Build history of the part. All positions in model axes, mm. Face numbers are marked on the shaded views. Give positions to 0.01 mm unless a question says otherwise; leave off trailing zeros. Loops run counter-clockwise (first coordinate to the right, second up) from the corner with the lowest first, then second, coordinate; pieces in that order, holes last. Notation, with made-up numbers: (80.5, 33) -> (87.5, 33) arc R28 cw to (87.5, 62) -> close; hole circle Ø10 at (31.5, 25). An arc over 180 degrees is marked (long way). One line per question, with ' | ' between items. Start each with the question number.
(1) Drill centre lines: L1, parallel to Y at x = -24, z = 6.5; L2, parallel to Y at x = -37.5, z = 11; L3, parallel to X at y = 22, z = 8.25. Where is each one in solid material? Low to high. Write a range as from..to.
(2) Mould opens along Y. For the marked faces 1, 2 and 3 say: pulls with the +Y half, pulls with the -Y half, needs draft (parallel to the pull), parting line crosses it, or undercut.
(3) Slice it at C-C, the plane y = 20. Write the cut outline in (x, z), then the cut area to 3 significant figures.
(4) Slice it at A-A, the plane z = 4.25. Write the cut outline in (x, y), then the cut area to 3 significant figures.
(5) Slice it at B-B, the plane x = -28.5. Write the cut outline in (y, z).
```python
from build123d import *

# Parameters (mm, degrees)
SKETCH1_W           = 50.8
SKETCH1_H           = 50.8
BOSS_EXTRUDE1_DEPTH = 14.478
SKETCH3_W           = 6.134078845
SKETCH3_H           = 10.131279463
SKETCH3_W_2         = 4.974615739
SKETCH3_H_2         = 3.542535777
SKETCH3_W_3         = 2.775050154
SKETCH3_H_3         = 5.132822303
SKETCH3_H_4         = 5.129144124
SKETCH3_W_4         = 11.43
SKETCH3_H_5         = 11.811
SKETCH3_W_5         = 4.097064437
SKETCH3_H_6         = 1.20756089
CUT_EXTRUDE1_DEPTH  = 13.97


with BuildPart() as part:
    # Sketch1 → Boss-Extrude1 (new body)
    with BuildSketch(Plane.XY):
        with Locations((-22.928187919, 27.871812081)):
            Rectangle(SKETCH1_W, SKETCH1_H)
    extrude(amount=BOSS_EXTRUDE1_DEPTH)

    # Sketch3 → Cut-Extrude1 (cut)
    with BuildSketch(Plane.XY.offset(14.478)):
        with Locations((-42.399843081, 34.61717235)):
            Rectangle(SKETCH3_W, SKETCH3_H)
        Polygon((-39.332803658, 27.871812081), (-34.358187919, 27.871812081), (-34.358187919, 39.682812081), (-39.332803658, 39.682812081), (-39.332803658, 29.551532618), align=None)
        Polygon((-22.928187919, 27.871812081), (-22.928187919, 39.682812081), (-27.293419188, 39.682812081), (-30.068469342, 39.682812081), (-34.358187919, 39.682812081), (-34.358187919, 27.871812081), align=None)
        Polygon((-17.868746746, 39.682812081), (-22.928187919, 39.682812081), (-22.928187919, 27.871812081), (-11.498187919, 27.871812081), (-11.498187919, 39.682812081), (-13.771682309, 39.682812081), align=None)
        Polygon((-22.928187919, 16.060812081), (-22.928187919, 27.871812081), (-34.358187919, 27.871812081), (-34.358187919, 24.329276304), (-34.358187919, 16.060812081), (-30.068469342, 16.060812081), (-27.293419188, 16.060812081), align=None)
        with Locations((-36.845495789, 26.100544193)):
            Rectangle(SKETCH3_W_2, SKETCH3_H_2)
        with Locations((-28.680944265, 13.49440093)):
            Rectangle(SKETCH3_W_3, SKETCH3_H_3)
        with Locations((-28.680944265, 42.247384143)):
            Rectangle(SKETCH3_W_3, SKETCH3_H_4)
        with Locations((-17.213187919, 21.966312081)):
            Rectangle(SKETCH3_W_4, SKETCH3_H_5)
        with Locations((-15.820214527, 40.286592526)):
            Rectangle(SKETCH3_W_5, SKETCH3_H_6)
    extrude(amount=-CUT_EXTRUDE1_DEPTH, mode=Mode.SUBTRACT)


solid = part.part
```
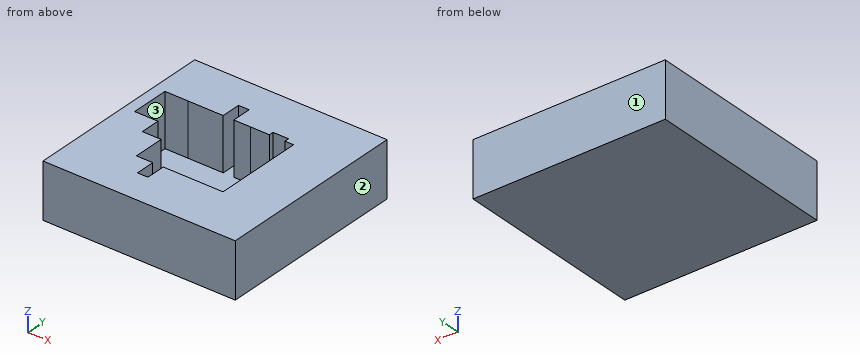
Final values:
1) L1: 2.47..16.06, 39.68..53.27 | L2: 2.47..24.33, 39.68..53.27 | L3: -48.33..-34.36, -11.5..2.47
2) face 1: pulls with the +Y half | face 2: needs draft | face 3: undercut
3) outline: (-48.33, 0) -> (2.47, 0) -> (2.47, 14.48) -> (-11.5, 14.48) -> (-11.5, 0.51) -> (-34.36, 0.51) -> (-34.36, 14.48) -> (-48.33, 14.48) -> close | area: 416 mm2
4) outline: (-48.33, 2.47) -> (2.47, 2.47) -> (2.47, 53.27) -> (-48.33, 53.27) -> close; hole (-45.47, 29.55) -> (-39.33, 29.55) -> (-39.33, 24.33) -> (-34.36, 24.33) -> (-34.36, 16.06) -> (-30.07, 16.06) -> (-30.07, 10.93) -> (-27.29, 10.93) -> (-27.29, 16.06) -> (-11.5, 16.06) -> (-11.5, 39.68) -> (-13.77, 39.68) -> (-13.77, 40.89) -> (-17.87, 40.89) -> (-17.87, 39.68) -> (-27.29, 39.68) -> (-27.29, 44.81) -> (-30.07, 44.81) -> (-30.07, 39.68) -> (-45.47, 39.68) -> close | area: 1,870 mm2
5) outline: (2.47, 0) -> (53.27, 0) -> (53.27, 14.48) -> (44.81, 14.48) -> (44.81, 0.51) -> (10.93, 0.51) -> (10.93, 14.48) -> (2.47, 14.48) -> close
